Can you work these out from the model? Positions are in its coordinate system, mm. Round coordinates to 2 decimals unless told otherwise and drop trailing zeros. Write each loop counter-clockwise with the first axis right and the second up, starting at its lowest first coordinate (ties: lowest second). Pieces come first, ordered by that corner, then holes. Notation, with made-up numbers: M -38.75,-15 L -5.75,-15 A20 ccw -5.75,-6 Z; hole C 73.5,12 d1. An arc over 180 degrees is marked long. Answer as a JSON object with one key per item and string values. Group by question number.
1) Suppose I cut it at C-C, the plane x = 4. Write out the boundary of the cut face in (y, z), and give its area (3 significant figures).
2) Please list where these lines run through material, in increasing order: L1, parallel to Y at x = 0, z = 2.5; L2, parallel to Y at x = -10, z = 2.25; L3, parallel to X at y = -4, z = 0.5. Write a range as [from, to].
3) Suppose I cut it at D-D, the plane y = -21.5. Write out the boundary of the cut face in (x, z).
4) Suppose I cut it at B-B, the plane y = 0. Write out the boundary of the cut face in (x, z).
5) Suppose I cut it at A-A, the plane z = 4.75. Write out the boundary of the cut face in (x, y), and give its area (3 significant figures).
6) I'm going to push flat-ended pins straight in: pin 1 Ø5 at (y, z) = (-12.5, 2.5) entering from +X; pin 2 Ø2 at (x, z) = (-15, 6) entering from +Y; pin 3 Ø5 at (y, z) = (20.5, 7.5) entering from +X. Where does each tip first touch, or does it pass through?
7) If we mould it in two halves opening along X, with no side actions, what happens to faces 1 (the cylindrical face through (16.453, 5.181, 5.07)), 2 (the flat face through (-9.81, 22.86, 5.07)), 3 (the flat face through (22.71, -10.15, 5.07))? For each: +X half, -X half, draft (parallel to the pull), parting line (faces both ways), or undercut.
from build123d import *

# Parameters (mm, degrees)
F0_R     = 27
F1_DEPTH = 10
F2_R     = 17.25
F3_DEPTH = 25
F5_DEPTH = 25


with BuildPart() as f1:
    # F0 (on Top) → F1 (new body)
    with BuildSketch(Plane.XY):
        Circle(F0_R)
    extrude(amount=F1_DEPTH)

    # F2 (on face) → F3 (cut)
    with BuildSketch(Plane.XY.offset(10)):
        Circle(F2_R)
    extrude(amount=-F3_DEPTH, mode=Mode.SUBTRACT)

    # F4 (on face) → F5 (cut)
    with BuildSketch(Plane.XY.offset(10)):
        with BuildLine():
            Line((-26.9902284894, -0.7263374486), (-19.3469779437, 18.8333333333))
            ThreePointArc((-19.3469779437, 18.8333333333), (-25.1481481481, 9.8270364159), (-26.9902284894, -0.7263374486))
        make_face()
        with BuildLine():
            Line((-19.3469779437, 18.8333333333), (0, 27))
            ThreePointArc((0, 27), (-10.5, 24.8746859277), (-19.3469779437, 18.8333333333))
        make_face()
        with BuildLine():
            ThreePointArc((19.3469779437, 18.8333333333), (10.5, 24.8746859277), (0, 27))
            Line((0, 27), (19.3469779437, 18.8333333333))
        make_face()
        with BuildLine():
            ThreePointArc((27, 0), (25.0136803018, 10.1644378969), (19.3469779437, 18.8333333333))
            Line((19.3469779437, 18.8333333333), (26.9902284894, -0.7263374486))
            ThreePointArc((26.9902284894, -0.7263374486), (26.9975570118, -0.3632015871), (27, 0))
        make_face()
        with BuildLine():
            ThreePointArc((18.3060568625, -19.8466189097), (24.5832190215, -11.1653635203), (26.9902284894, -0.7263374486))
            Line((26.9902284894, -0.7263374486), (18.3060568625, -19.8466189097))
        make_face()
        with BuildLine():
            ThreePointArc((0, -27), (9.8270364159, -25.1481481481), (18.3060568625, -19.8466189097))
            Line((18.3060568625, -19.8466189097), (0, -27))
        make_face()
        with BuildLine():
            Line((0, -27), (-18.3060568625, -19.8466189097))
            ThreePointArc((-18.3060568625, -19.8466189097), (-9.8270364159, -25.1481481481), (0, -27))
        make_face()
        with BuildLine():
            Line((-18.3060568625, -19.8466189097), (-26.9902284894, -0.7263374486))
            ThreePointArc((-26.9902284894, -0.7263374486), (-24.5832190215, -11.1653635203), (-18.3060568625, -19.8466189097))
        make_face()
    extrude(amount=-F5_DEPTH, mode=Mode.SUBTRACT)


solid = f1.part
Results:
{
 "1": {"outline": "M -25.44,0 L -16.78,0 L -16.78,10 L -25.44,10 Z; M 16.78,0 L 25.31,0 L 25.31,10 L 16.78,10 Z", "area": "172 mm^2"},
 "2": {"L1": "[-27, -17.25], [17.25, 27]", "L2": "[-23.09, -14.06], [14.06, 22.78]", "L3": "[-25.5, -16.78], [16.78, 25.5]"},
 "3": {"outline": "M -14.07,0 L 14.07,0 L 14.07,10 L -14.07,10 Z"},
 "4": {"outline": "M -26.71,0 L -17.25,0 L -17.25,10 L -26.71,10 Z; M 17.25,0 L 26.71,0 L 26.71,10 L 17.25,10 Z"},
 "5": {"outline": "M -26.99,-0.73 L -18.31,-19.85 L 0,-27 L 18.31,-19.85 L 26.99,-0.73 L 19.35,18.83 L 0,27 L -19.35,18.83 Z; hole C 0,0 d34.5", "area": "1,130 mm^2"},
 "6": {"pin 1": "x = 22.78", "pin 2": "y = 21.09", "pin 3": "x = 19.67"},
 "7": {"face 1": "undercut", "face 2": "-X half", "face 3": "+X half"}
}
